from build123d import *

# Parameters (mm, degrees)
CROQUIS1_W                   = 15
CROQUIS1_H                   = 24
SALIENTE_EXTRUIR1_DEPTH      = 32.5
SALIENTE_EXTRUIR1_DEPTH_BACK = 32.5
CORTAR_EXTRUIR1_DEPTH        = 65.5
CORTAR_EXTRUIR2_DEPTH        = 65.5
SALIENTE_EXTRUIR2_DEPTH      = 3
CROQUIS5_R                   = 3.1
CORTAR_EXTRUIR3_DEPTH        = 3
CROQUIS6_R                   = 6.5
CORTAR_EXTRUIR5_DEPTH        = 2.5
CROQUIS7_W                   = 12
CROQUIS7_H                   = 14.5
SALIENTE_EXTRUIR3_DEPTH      = 1.5
CROQUIS8_R                   = 6
CROQUIS8_R_2                 = 3.5
SALIENTE_EXTRUIR4_DEPTH      = 3
CORTAR_EXTRUIR6_DEPTH        = 2
CROQUIS10_R                  = 1.5
CORTAR_EXTRUIR7_DEPTH        = 2
CROQUIS11_R                  = 3
CORTAR_EXTRUIR8_DEPTH        = 2
CROQUIS12_R                  = 1.5
SALIENTE_EXTRUIR5_DEPTH      = 2


with BuildPart() as part:
    # Croquis1 → Saliente-Extruir1 (new body, two sides)
    with BuildSketch(Plane(origin=(0, 0, 0), x_dir=(0, 0, -1), z_dir=(1, 0, 0))) as saliente_extruir1_sk:
        Rectangle(CROQUIS1_W, CROQUIS1_H)
    extrude(amount=SALIENTE_EXTRUIR1_DEPTH)
    extrude(saliente_extruir1_sk.sketch, amount=-SALIENTE_EXTRUIR1_DEPTH_BACK)

    # Croquis2 → Cortar-Extruir1 (cut)
    with BuildSketch(Plane(origin=(32.5, 0, 0), x_dir=(0, 0, -1), z_dir=(1, 0, 0))):
        Polygon((-7.5, 11), (-6.5, 11), (-6.5, 10), (-7, 10), (-7, -12), (-7.5, -12), align=None)
    extrude(amount=-CORTAR_EXTRUIR1_DEPTH, mode=Mode.SUBTRACT)

    # Croquis3 → Cortar-Extruir2 (cut)
    with BuildSketch(Plane(origin=(32.5, 0, 0), x_dir=(0, 0, -1), z_dir=(1, 0, 0))):
        Polygon((7.5, 11), (6.5, 11), (6.5, 10), (-4, 10), (-4, -10), (7.5, -10), align=None)
    extrude(amount=-CORTAR_EXTRUIR2_DEPTH, mode=Mode.SUBTRACT)

    # Croquis4 → Saliente-Extruir2 (add)
    with BuildSketch(Plane.XY.offset(7)):
        with BuildLine():
            Line((-3.553211575, 3.553211575), (-4.260318357, 4.260318357))
            ThreePointArc((-4.260318357, 4.260318357), (0, 6.025), (4.260318357, 4.260318357))
            Line((4.260318357, 4.260318357), (3.553211575, 3.553211575))
            ThreePointArc((3.553211575, 3.553211575), (0, 5.025), (-3.553211575, 3.553211575))
        make_face()
        with BuildLine():
            Line((-1.922984248, -4.642494651), (-2.30566768, -5.566374183))
            ThreePointArc((-2.30566768, -5.566374183), (0, -6.025), (2.30566768, -5.566374183))
            Line((2.30566768, -5.566374183), (1.922984248, -4.642494651))
            ThreePointArc((1.922984248, -4.642494651), (0, -5.025), (-1.922984248, -4.642494651))
        make_face()
    extrude(amount=SALIENTE_EXTRUIR2_DEPTH)

    # Croquis5 → Cortar-Extruir3 (cut)
    with BuildSketch(Plane.XY.offset(7)):
        Circle(CROQUIS5_R)
    extrude(amount=-CORTAR_EXTRUIR3_DEPTH, mode=Mode.SUBTRACT)

    # Croquis6 → Cortar-Extruir5 (cut)
    with BuildSketch(Plane(origin=(0, 0, 4), x_dir=(-1, 0, 0), z_dir=(0, 0, -1))):
        Circle(CROQUIS6_R)
    extrude(amount=-CORTAR_EXTRUIR5_DEPTH, mode=Mode.SUBTRACT)

    # Croquis7 → Saliente-Extruir3 (add)
    with BuildSketch(Plane.XZ.offset(12)):
        with Locations((0, -0.25)):
            Rectangle(CROQUIS7_W, CROQUIS7_H)
    extrude(amount=SALIENTE_EXTRUIR3_DEPTH)

    # Croquis8 → Saliente-Extruir4 (add)
    with BuildSketch(Plane.XZ.offset(13.5)):
        Circle(CROQUIS8_R)
        Circle(CROQUIS8_R_2, mode=Mode.SUBTRACT)
    extrude(amount=SALIENTE_EXTRUIR4_DEPTH)

    # Croquis9 → Cortar-Extruir6 (cut)
    with BuildSketch(Plane(origin=(0, -10, 0), x_dir=(1, 0, 0), z_dir=(0, 1, 0))):
        with BuildLine():
            Line((3, 7.5), (-3, 7.5))
            Line((-3, 7.5), (-3, 0.5))
            ThreePointArc((-3, 0.5), (0, -2.5), (3, 0.5))
            Line((3, 0.5), (3, 7.5))
        make_face()
    extrude(amount=-CORTAR_EXTRUIR6_DEPTH, mode=Mode.SUBTRACT)

    # Croquis10 → Cortar-Extruir7 (cut)
    with BuildSketch(Plane.XZ.offset(13.5)):
        Circle(CROQUIS10_R)
    extrude(amount=-CORTAR_EXTRUIR7_DEPTH, mode=Mode.SUBTRACT)

    # Croquis11 → Cortar-Extruir8 (cut)
    with BuildSketch(Plane(origin=(0, 12, 0), x_dir=(1, 0, 0), z_dir=(0, 1, 0))):
        Circle(CROQUIS11_R)
    extrude(amount=-CORTAR_EXTRUIR8_DEPTH, mode=Mode.SUBTRACT)

    # Croquis12 → Saliente-Extruir5 (add)
    with BuildSketch(Plane.XZ.offset(12)):
        with BuildLine():
            Line((32.5, -10), (32.5, 10))
            ThreePointArc((32.5, 10), (29, 13.5), (25.5, 10))
            Line((25.5, 10), (25.5, -10))
            ThreePointArc((25.5, -10), (29, -13.5), (32.5, -10))
        make_face()
        with Locations((29, 10)):
            Circle(CROQUIS12_R, mode=Mode.SUBTRACT)
        with Locations((29, -10)):
            Circle(CROQUIS12_R, mode=Mode.SUBTRACT)
        with BuildLine():
            Line((-25.5, -10), (-25.5, 10))
            ThreePointArc((-25.5, 10), (-29, 13.5), (-32.5, 10))
            Line((-32.5, 10), (-32.5, -10))
            ThreePointArc((-32.5, -10), (-29, -13.5), (-25.5, -10))
        make_face()
        with Locations((-29, 10)):
            Circle(CROQUIS12_R, mode=Mode.SUBTRACT)
        with Locations((-29, -10)):
            Circle(CROQUIS12_R, mode=Mode.SUBTRACT)
    extrude(amount=SALIENTE_EXTRUIR5_DEPTH)


solid = part.part
Can you work these out from the model? Positions are in its coordinate system, mm. A direction names the side the tool comes from. Give positions to 0.01 mm unless a question says otherwise; leave off trailing zeros. Write each loop counter-clockwise with the first axis right and the second up, starting at its lowest first coordinate (ties: lowest second). Pieces come first, ordered by that corner, then holes. Notation, with made-up numbers: M 27,79 L 33,79 A29 ccw 33,115 Z; hole C -35,-7 d7. An arc over 180 degrees is marked long. Answer in a Markdown table with one row per item. Add a question column.
Item 1: On a 3-axis mill with a long thin cutter (end or side, diameter ignored), from which of +Z, -Z, +X, -X, +Y, -Y can I reach the whole of each face in a straight line? I mean faces 1 (the flat face through (0, -13.5, -2)), 2 (the flat face through (-29, -14, 0)), 3 (the cylindrical face through (0.028, -5.025, 8.479)), 4 (the flat face through (0, -10, 3)), 5 (the flat face through (31, -12, -10)). Say none if no direction works.
Item 2: Imagine slicing it at A-A, the plane x = -18. Write out the boundary of the cut face in (y, z).
Item 3: Imagine slicing it at D-D, the plane y = -9. Write out the boundary of the cut face in (x, z), plus the area to 3 significant figures.
Item 4: Imagine slicing it at C-C, the plane x = 0. State how many separate pieces and enclosed holes the cut face has, plus the area to 4 significant figures.
Item 5: For pin 1 Ø7 at (x, y) = (0, 0) entering from -Z; pin 2 Ø4 at (x, z) = (-10.5, -1) entering from -Y; pin 3 Ø3 at (x, z) = (28, -10.5) entering from +Y, each with a flat end and sliding along its axis, tell me the tip position at first contact or that it passes through.
Item 6: We'd pull the mould along X, two halves only. Please class faces 6 (the flat face through (-3, -11, -4)), 7 (the flat face through (32.5, -2.9, 4.4)), 8 (the flat face through (27, -12, 10)): released by +X, released by -X, zero draft, split by the parting line, or undercut.
Item 7: Please list where these lines run through material, in increasing order: L1, parallel to Z at x = 29, y = -13.25; L2, parallel to Y at x = -21.5, z = 1.5; L3, parallel to Z at x = 0, y = 10.9.
Item 8: Imagine slicing it at B-B, the plane z = -4.25. Write out the boundary of the cut face in (x, y).
Evaluation:
| question | item | result |
|---|---|---|
| 1 | face 1 | -Y |
| 1 | face 2 | +Z, -Z, -X, -Y |
| 1 | face 3 | +Z |
| 1 | face 4 | -Z, +X, -X |
| 1 | face 5 | -Z, +X, -X, +Y |
| 2 | outline | M -12,-7.5 L -10,-7.5 L -10,4 L 10,4 L 10,-6.5 L 11,-6.5 L 11,-7.5 L 12,-7.5 L 12,7.5 L 11,7.5 L 11,6.5 L 10,6.5 L 10,7 L -12,7 Z |
| 3 | outline | M -32.5,4 L 32.5,4 L 32.5,7 L -32.5,7 Z |
| 3 | area | 195 mm² |
| 4 | separate pieces | 4 |
| 4 | enclosed holes | 0 |
| 4 | area | 87.65 mm² |
| 5 | pin 1 | stops at z = 6.5 |
| 5 | pin 2 | stops at y = -12 |
| 5 | pin 3 | stops at y = -12 |
| 6 | face 6 | undercut |
| 6 | face 7 | released by +X |
| 6 | face 8 | zero draft |
| 7 | L1 | z = -13.5 to -11.5, -8.5 to 8.5, 11.5 to 13.5 |
| 7 | L2 | y = -12 to -10, 10 to 12 |
| 7 | L3 | z = -6.5 to -3, 3 to 6.5 |
| 8 | outline | M -32.5,-14 L -25.5,-14 L -25.5,-12 L -6,-12 L -6,-13.5 L -4.24,-13.5 L -4.24,-16.5 L 4.24,-16.5 L 4.24,-13.5 L 6,-13.5 L 6,-12 L 25.5,-12 L 25.5,-14 L 32.5,-14 L 32.5,-10 L 3,-10 L 3,-12 L -3,-12 L -3,-10 L -32.5,-10 Z; M -32.5,10 L 32.5,10 L 32.5,12 L -32.5,12 Z |
